```python
from build123d import *

# Parameters (mm, degrees)
SKETCH_1_W           = 5
SKETCH_1_H           = 30
EXTRUDE_1_DEPTH      = 5
EXTRUDE_2_DEPTH      = 20
EXTRUDE_2_DEPTH_BACK = 5
SKETCH_1_3_W         = 5
SKETCH_1_3_H         = 30
SKETCH_3_R           = 4
CUT_EXTRUDE_2_DEPTH  = 57.844085005
SKETCH_5_W           = 11
SKETCH_5_H           = 15
CUT_EXTRUDE_3_DEPTH  = 10


with BuildPart() as part:
    # Sketch 1 → Extrude 1 (new body)
    with BuildSketch(Plane(origin=(0, 0, 0), x_dir=(0, 0, -1), z_dir=(1, 0, 0))):
        Polygon((17.5, 27.5), (-17.5, 27.5), (-17.5, -2.5), (-22.5, -2.5), (-22.5, -27.5), (22.5, -27.5), (22.5, -2.5), (17.5, -2.5), align=None)
        with Locations((-20, 12.5)):
            Rectangle(SKETCH_1_W, SKETCH_1_H)
        with BuildLine():
            Line((-22.5, 27.5), (-17.5, 27.5))
            ThreePointArc((-17.5, 27.5), (0, 45), (17.5, 27.5))
            Line((17.5, 27.5), (22.5, 27.5))
            ThreePointArc((22.5, 27.5), (0, 50), (-22.5, 27.5))
        make_face()
        with BuildLine():
            ThreePointArc((17.5, 27.5), (0, 45), (-17.5, 27.5))
            Line((-17.5, 27.5), (17.5, 27.5))
        make_face()
        with Locations((20, 12.5)):
            Rectangle(SKETCH_1_W, SKETCH_1_H)
    extrude(amount=EXTRUDE_1_DEPTH)

    # Sketch 1_3 → Extrude 2 (add, two sides: drawn at the far end of the back side and taken through both)
    with BuildSketch(Plane(origin=(0, 0, 0), x_dir=(0, 0, -1), z_dir=(1, 0, 0)).offset(-EXTRUDE_2_DEPTH_BACK)):
        with BuildLine():
            Line((-22.5, 27.5), (-17.5, 27.5))
            ThreePointArc((-17.5, 27.5), (0, 45), (17.5, 27.5))
            Line((17.5, 27.5), (22.5, 27.5))
            ThreePointArc((22.5, 27.5), (0, 50), (-22.5, 27.5))
        make_face()
        with Locations((-20, 12.5)):
            Rectangle(SKETCH_1_3_W, SKETCH_1_3_H)
        with Locations((20, 12.5)):
            Rectangle(SKETCH_1_3_W, SKETCH_1_3_H)
    extrude(amount=EXTRUDE_2_DEPTH + EXTRUDE_2_DEPTH_BACK)

    # Sketch 3 → Cut-Extrude 2 (cut, through all)
    with BuildSketch(Plane(origin=(5, 0, 0), x_dir=(0, 0, -1), z_dir=(1, 0, 0))):
        with Locations((-13.5, -19.5)):
            Circle(SKETCH_3_R)
        with Locations((13.5, -19.5)):
            Circle(SKETCH_3_R)
        Circle(SKETCH_3_R)
    extrude(amount=-CUT_EXTRUDE_2_DEPTH, mode=Mode.SUBTRACT)

    # Sketch 5 → Cut-Extrude 3 (cut)
    with BuildSketch(Plane(origin=(20, 0, 0), x_dir=(0, 0, -1), z_dir=(1, 0, 0))):
        with Locations((0, 47.5)):
            Rectangle(SKETCH_5_W, SKETCH_5_H)
    extrude(amount=-CUT_EXTRUDE_3_DEPTH, mode=Mode.SUBTRACT)


solid = part.part
```
Input: part model. Units: mm. Frame: model coordinates. A direction names the side the tool comes from. Round coordinates to 2 decimals unless told otherwise and drop trailing zeros. Write each loop counter-clockwise with the first axis right and the second up, starting at its lowest first coordinate (ties: lowest second). Pieces come first, ordered by that corner, then holes. Notation, with made-up numbers: M 89,58 L 102,58 A17 cw 102,72 Z; hole C 69,-1.5 d9. An arc over 180 degrees is marked long. Write each question's results on one line, items separated by ' | '.
Q1. Section query D-D (y = 8). Return loops of the section in (x, z).
Results:
outline: M -5,-22.5 L 20,-22.5 L 20,-17.5 L 5,-17.5 L 5,17.5 L 20,17.5 L 20,22.5 L -5,22.5 L -5,17.5 L 0,17.5 L 0,-17.5 L -5,-17.5 Z
Q2. Access query for faces 4 (the face through (-3, -2.5, -20)), 5 (the face through (7, 50, 0)), 6 (the face through (12, -2.5, -20)), 7 (the face through (-3, 45, 0)), 8 (the face through (12, 12, 17.5)). Directions: +Z, -Z, +X, -X, +Y, -Y. A direction counts if a zero-diameter tool reaches every point of the face in a straight line with its end or side. Return the directions, or none.
Results:
face 4: +Z, -Z, -X, -Y | face 5: +X, -X, +Y | face 6: +Z, -Z, +X, -Y | face 7: -X, -Y | face 8: +X, -Y
Q3. Line query: line 1 along Z through (x, y) = (-2.25, 20); line 2 along Y through (x, z) = (1.95, 0); line 3 along X through (y, z) = (-9, 0.5). Output: solid intervals per line, ascending.
Results:
line 1: z = -22.5 to -17.5, 17.5 to 22.5 | line 2: y = -27.5 to -4, 4 to 50 | line 3: x = 0 to 5
Q4. Section query C-C (y = 0). Return loops of the section in (x, z).
Results:
outline: M -5,-22.5 L 20,-22.5 L 20,-17.5 L 5,-17.5 L 5,-4 L 0,-4 L 0,-17.5 L -5,-17.5 Z; M -5,17.5 L 0,17.5 L 0,4 L 5,4 L 5,17.5 L 20,17.5 L 20,22.5 L -5,22.5 Z
Q5. Draft query along Y for faces 1 (the face through (2.535, -3.905, 0.867)), 2 (the face through (7, 6, 22.5)), 3 (the face through (12, -2.5, 20)). Return one class per face: released by +Y, released by -Y, zero draft, split by the parting line, or undercut.
Results:
face 1: undercut | face 2: zero draft | face 3: released by -Y
Q6. Section query A-A (y = -19.5). Return loops of the section in (x, z).
Results:
outline: M 0,-22.5 L 5,-22.5 L 5,-17.5 L 0,-17.5 Z; M 0,-9.5 L 5,-9.5 L 5,9.5 L 0,9.5 Z; M 0,17.5 L 5,17.5 L 5,22.5 L 0,22.5 Z
Q7. Section query B-B (x = 12.5). Return loops of the section in (y, z), and give its area (3 significant figures).
Results:
outline: M -2.5,-22.5 L 27.5,-22.5 A22.5 ccw 49.32,-5.5 L 44.11,-5.5 A17.5 cw 27.5,-17.5 L -2.5,-17.5 Z; M -2.5,17.5 L 27.5,17.5 A17.5 cw 44.11,5.5 L 49.32,5.5 A22.5 ccw 27.5,22.5 L -2.5,22.5 Z | area: 558 mm^2
Q8. Pin query (flat end, axial travel): P1, Ø7, axis at y = -19.5, z = 13.5, coming from the +X side; P2, Ø3, axis at x = 9, z = 3, coming from the +Y side; P3, Ø12, axis at x = 9, y = 32, coming from the +Z side; P4, Ø8, axis at y = -12.5, z = -1.5, coming from the -X side. Return the tip coordinate at first contact, or that it passes through.
Results:
P1: passes through | P2: stops at y = 49.95 | P3: stops at z = 22.5 | P4: stops at x = 0
